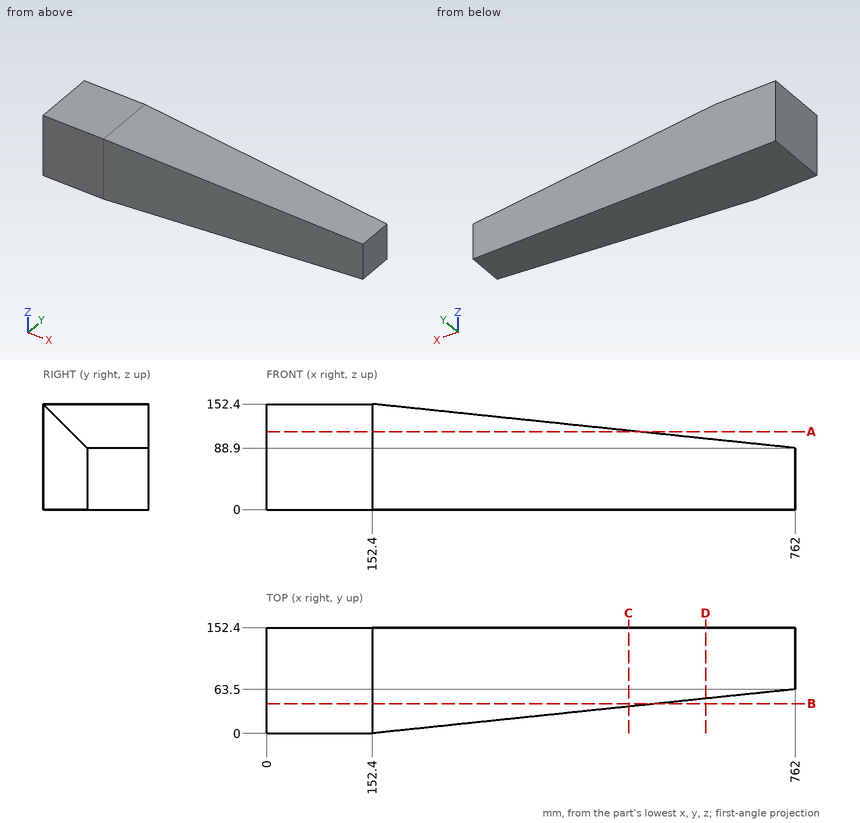
Print and shaded views of the part. All mm, measured from the part's lowest x, y and z. Give positions to 0.01 mm unless a question says otherwise; leave off trailing zeros. Write each loop counter-clockwise with the first axis right and the second up, starting at its lowest first coordinate (ties: lowest second). Pieces come first, ordered by that corner, then holes. Notation, with made-up numbers: (44.25, -37) -> (68.25, -37) arc R20 cw to (68.25, -24) -> close; hole circle Ø3 at (89, 53.5). An arc over 180 degrees is marked (long way). Use CSV: the item, a comma, the result in double quotes. Start each with the question number.
1) Drill centre lines: L1, parallel to Z at x = 407.5, y = 45.5; L2, parallel to Z at x = 340.5, y = 38.5; L3, parallel to Y at x = 584.5, z = 50. Where is each one in solid material? Low to high.
2) Cut at D-D on x = 633. List the corners of the cut face in (y, z), plus the area to 3 significant figures.
3) Cut at C-C on x = 522. List the corners of the cut face in (y, z), plus the area to 3 significant figures.
4) Cut at A-A on z = 112.5. List the corners of the cut face in (x, y).
5) Cut at B-B on y = 43. List the corners of the cut face in (x, z).
6) Pin check, flat tips, straight feed: P1, Ø10, axis at x = 555, y = 68.5, coming from the +Z side; P2, Ø1.5, axis at x = 524, z = 24, coming from the -Y side. Stop position of each tip, or through.
Final values:
1,L1,"z = 0 to 125.83"
1,L2,"z = 0 to 132.81"
1,L3,"y = 45.01 to 152.4"
2,outline,"(50.06, 0) -> (152.4, 0) -> (152.4, 102.34) -> (50.06, 102.34) -> close"
2,area,"10,500 mm2"
3,outline,"(38.5, 0) -> (152.4, 0) -> (152.4, 113.9) -> (38.5, 113.9) -> close"
3,area,"13,000 mm2"
4,outline,"(0, 0) -> (152.4, 0) -> (535.44, 39.9) -> (535.44, 152.4) -> (0, 152.4) -> close"
5,outline,"(0, 0) -> (565.2, 0) -> (565.2, 109.4) -> (152.4, 152.4) -> (0, 152.4) -> close"
6,P1,"stops at z = 110.98"
6,P2,"stops at y = 38.63"
